Source: CAD feature listing. Evaluate the final solid. Frame: model axes, mm. A direction names the side the tool comes from. Give positions to 0.01 mm unless a question says otherwise; leave off trailing zeros. Order: outer loops, then holes, each group sorted by start corner. A loop starts at its lowest first (then second) coordinate and runs counter-clockwise, first axis right, second up. Notation, with made-up numbers: M -31.5,-2.5 L -22.5,-2.5 A20 cw -22.5,3.5 Z; hole C 7.25,74.5 d1. An arc over 180 degrees is marked long. Return JSON: item names as keys, results as strings.
from build123d import *

# Parameters (mm, degrees)
CYLINDER006_R     = 0.25
CYLINDER006_DEPTH = 8
CYLINDER007_R     = 0.25
CYLINDER007_DEPTH = 8
CYLINDER008_R     = 0.25
CYLINDER008_DEPTH = 8
CYLINDER009_R     = 0.25
CYLINDER009_DEPTH = 8
CYLINDER005_R     = 4.5
CYLINDER005_DEPTH = 8


with BuildPart() as cylinder006:
    # Cylinder006 → Cylinder006 (new body)
    with BuildSketch(Plane(origin=(6, 15, 0), x_dir=(1, 0, 0), z_dir=(0, 0, 1))):
        Circle(CYLINDER006_R)
    extrude(amount=CYLINDER006_DEPTH)


with BuildPart() as cylinder007:
    # Cylinder007 → Cylinder007 (new body)
    with BuildSketch(Plane(origin=(6, 19, 0), x_dir=(1, 0, 0), z_dir=(0, 0, 1))):
        Circle(CYLINDER007_R)
    extrude(amount=CYLINDER007_DEPTH)


with BuildPart() as cylinder008:
    # Cylinder008 → Cylinder008 (new body)
    with BuildSketch(Plane(origin=(10, 19, 0), x_dir=(1, 0, 0), z_dir=(0, 0, 1))):
        Circle(CYLINDER008_R)
    extrude(amount=CYLINDER008_DEPTH)


with BuildPart() as cylinder009:
    # Cylinder009 → Cylinder009 (new body)
    with BuildSketch(Plane(origin=(10, 15, 0), x_dir=(1, 0, 0), z_dir=(0, 0, 1))):
        Circle(CYLINDER009_R)
    extrude(amount=CYLINDER009_DEPTH)


with BuildPart() as capacitor:
    # Cylinder005 → Cylinder005 (new body)
    with BuildSketch(Plane(origin=(8, 17, 8), x_dir=(1, 0, 0), z_dir=(0, 0, 1))):
        Circle(CYLINDER005_R)
    extrude(amount=CYLINDER005_DEPTH)

    # Fusion001: union Cylinder006, Cylinder007, Cylinder008, Cylinder009
    add(cylinder006.part)
    add(cylinder007.part)
    add(cylinder008.part)
    add(cylinder009.part)


solid = capacitor.part
1. Ray query, probe 1 along Z at (x, y) = (5.5, 18.5); probe 2 along X at (y, z) = (21, 8.5); probe 3 along X at (y, z) = (15.75, 11.5). Return the intervals inside material, ascending.
Evaluation:
{"probe 1": "z = 8 to 16", "probe 2": "x = 5.94 to 10.06", "probe 3": "x = 3.68 to 12.32"}
2. First-contact query: pin 1 (1.5 mm diameter, centred on x = 11.5, y = 20.5, fed in from -Z); pin 2 (1 mm diameter, centred on x = 6.5, z = 2.5, fed in from -Y); pin 3 (2 mm diameter, centred on y = 18.5, z = 5.5, fed in from +X). Flat tips, straight axial feed; report the tip coordinate or a pass-through.
Evaluation:
{"pin 1": "stops at z = 8", "pin 2": "stops at y = 14.75", "pin 3": "stops at x = 10.25"}
3. Section query A-A (x = 6). Return loops of the section in (y, z).
Evaluation:
{"outline": "M 12.97,8 L 14.75,8 L 14.75,0 L 15.25,0 L 15.25,8 L 18.75,8 L 18.75,0 L 19.25,0 L 19.25,8 L 21.03,8 L 21.03,16 L 12.97,16 Z"}
4. Section query D-D (z = 12). Return loops of the section in (x, y).
Evaluation:
{"outline": "C 8,17 d9"}
5. Section query B-B (z = 7.5). Return loops of the section in (x, y), then the cut area to 3 significant figures.
Evaluation:
{"outline": "C 6,15 d0.5; C 6,19 d0.5; C 10,15 d0.5; C 10,19 d0.5", "area": "0.785 mm^2"}
6. Section query C-C (y = 17). Return loops of the section in (x, z).
Evaluation:
{"outline": "M 3.5,8 L 12.5,8 L 12.5,16 L 3.5,16 Z"}
7. Set-up query: faces 1 (the face through (8, 17, 8)), 2 (the face through (10.419, 20.794, 11.944)). Return all of +Z, -Z, +X, -X, +Y, -Y with unobstructed straight access to the full face (end or side cutting, diameter ignored); none if empty.
Evaluation:
{"face 1": "-Z", "face 2": "+Z, -Z"}
